For this review, use the dimensioned drawing (mm, ordinates from the lowest corner) and the shaded views. A direction names the side the tool comes from. Give positions to 0.01 mm unless a question says otherwise; leave off trailing zeros. Write each loop counter-clockwise with the first axis right and the second up, starting at its lowest first coordinate (ties: lowest second). Pieces come first, ordered by that corner, then holes. Notation, with made-up numbers: (40.25, -11) - (45.25, -11) arc R33 ccw to (45.25, 24) - close; hole circle Ø4 at (-16, 24.25). An arc over 180 degrees is marked (long way). One line per question, with ' | ' between items. Start each with the question number.
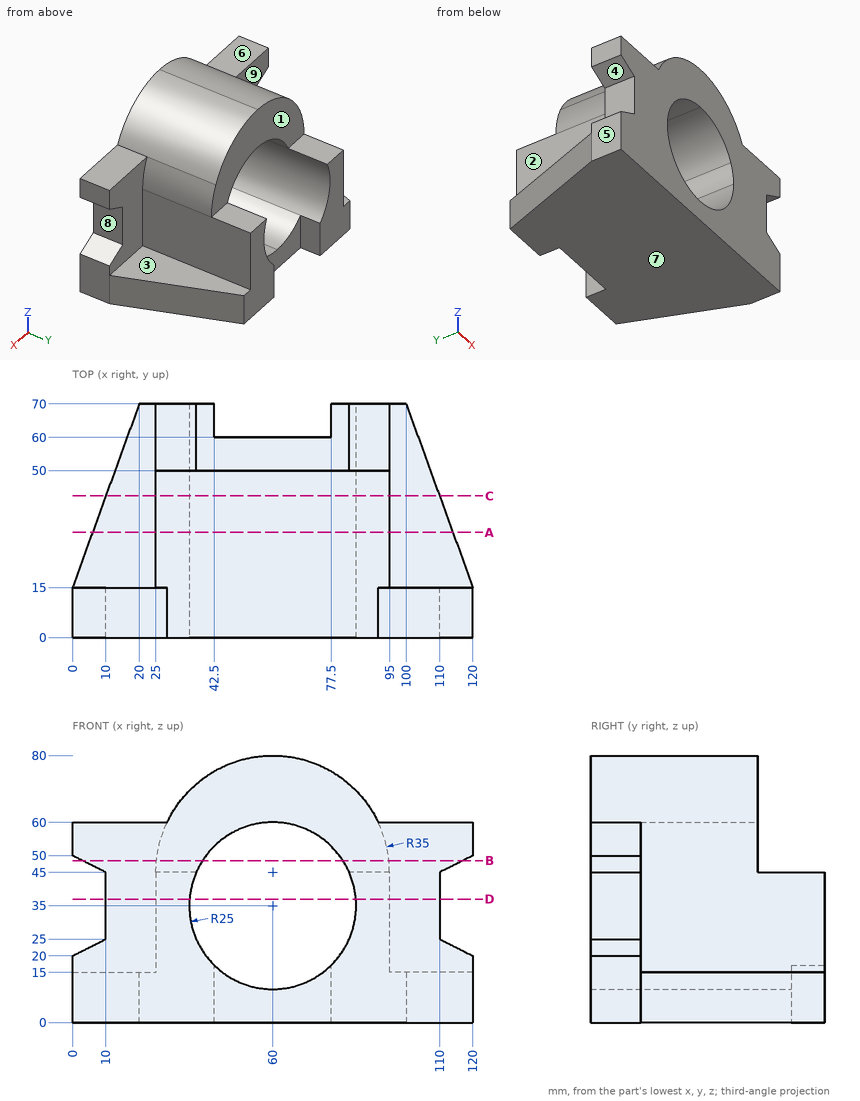
Item 1: Take a section at D-D (z = 37). Give the boundary of the cut face in (x, y).
Item 2: Machinability: for the marked faces 1, 2, 3, 4 and 5, which of the approach directions +Z, -Z, +X, -X, +Y, -Y give a long, thin tool a straight path to every point of the face, cutting with its end or side? Answer none if there is none.
Item 3: Clearance check with flat-ended pins moving along their axes: P1, Ø7.5, axis at x = 105, y = 43.5, coming from the +Z side; P2, Ø3, axis at y = 66.5, z = 6.5, coming from the -X side; P3, Ø9.5, axis at x = 29.5, y = 55.5, coming from the +Z side; P4, Ø2, axis at x = 33, z = 41.5, coming from the -Y side. State where each tip first meets the part, or that it passes through.
Item 4: Take a section at A-A (y = 31.5). Give the boundary of the cut face in (x, z), plus the area to 3 significant figures.
Item 5: Take a section at B-B (z = 48.5). Give the boundary of the cut face in (x, y), plus the area to 3 significant figures.
Item 6: Take a section at C-C (y = 42.5). Give the boundary of the cut face in (x, z).
Item 7: For probe 1 along Z at (x, y) = (18, 32); probe 2 along Y at (x, z) = (43, 13), list the stretches that pass through material, from the lowest coordinate up.
Item 8: The part is to be moulded in two halves that separate along Z. For the marked faces 6, 7, 8 and 9, say which applies: +Z half, -Z half, draft (parallel to the pull), parting line (faces both ways), or undercut.
Check sheet entries:
1) outline: (10, 0) - (35.08, 0) - (35.08, 70) - (25, 70) - (25, 15) - (10, 15) - close; (84.92, 0) - (110, 0) - (110, 15) - (95, 15) - (95, 70) - (84.92, 70) - close
2) face 1: +Z, +X, -X, +Y | face 2: +Z, -X, +Y | face 3: +Z, +X, +Y | face 4: -X, +Y, -Y | face 5: +Z, -Z, -X, +Y, -Y
3) P1: stops at z = 15 | P2: stops at x = 18.18 | P3: stops at z = 45 | P4: stops at y = 0
4) outline: (6, 0) - (114, 0) - (114, 15) - (95, 15) - (95, 45) arc R35 ccw to (25, 45) - (25, 15) - (6, 15) - close; hole circle Ø50 at (60, 35) | area: 3,680 mm^2
5) outline: (3, 0) - (38.96, 0) - (38.96, 50) - (25.18, 50) - (25.18, 15) - (3, 15) - close; (81.04, 0) - (117, 0) - (117, 15) - (94.82, 15) - (94.82, 50) - (81.04, 50) - close | area: 2,040 mm^2
6) outline: (10, 0) - (110, 0) - (110, 15) - (95, 15) - (95, 45) arc R35 ccw to (25, 45) - (25, 15) - (10, 15) - close; hole circle Ø50 at (60, 35)
7) probe 1: z = 0 to 15 | probe 2: y = 0 to 60
8) face 6: +Z half | face 7: -Z half | face 8: undercut | face 9: draft
